Autodesk Inventor part; units mm, degrees
ref_plane "YZ Plane" through (0, 0, 0) normal (1, 0, 0) x (0, 1, 0)
ref_plane "XZ Plane" through (0, 0, 0) normal (0, 1, 0) x (-1, 0, 0)
ref_plane "XY Plane" through (0, 0, 0) normal (0, 0, 1) x (1, 0, 0)
sketch "Sketch1" plane through (0, 0, 0) normal (0, 1, 0) x (-1, 0, 0)
  line L0 (17.6552, 44.8276) -> (77.6552, 44.8276)
  line L1 (77.6552, 44.8276) -> (77.6552, -15.1724)
  line L2 (77.6552, -15.1724) -> (17.6552, -15.1724)
  line L3 (17.6552, -15.1724) -> (17.6552, 44.8276)
  point P0 (0, 0)
  dimension "d0" = 60
  dimension "d1" = 60
extrude "Extrusion1" add sketch "Sketch1" along normal blind 25
sketch "Sketch2" plane through (0, 25, 0) normal (0, 1, 0) x (1, 0, 0)
  line L0 (-17.6552, -44.8276) -> (-17.6552, 15.1724)
  line L1 (-17.6552, 15.1724) -> (-77.6552, 15.1724)
  line L2 (-77.6552, 15.1724) -> (-77.6552, -44.8276)
  circle A0 centre (-47.6552, -14.8276) radius 26
  circle A1 centre (-73.6552, 11.1724) radius 2.15
  circle A2 centre (-21.6552, 11.1724) radius 2.15
  circle A3 centre (-21.6552, -40.8276) radius 2.15
  circle A4 centre (-73.6552, -40.8276) radius 2.15
  point P0 (0, 0)
  dimension "d4" = 52
  dimension "d5" = 30
  dimension "d6" = 30
  dimension "d7" = 4.3
  dimension "d8" = 4.3
  dimension "d9" = 4.3
  dimension "d10" = 4.3
  dimension "d11" = 52
  dimension "d12" = 52
  dimension "d13" = 52
  dimension "d14" = 52
  dimension "d15" = 4
  dimension "d16" = 4
  dimension "d17" = 4
  dimension "d18" = 4
extrude "Extrusion2" cut sketch "Sketch2" against normal blind 38
properties part number "Fan60"
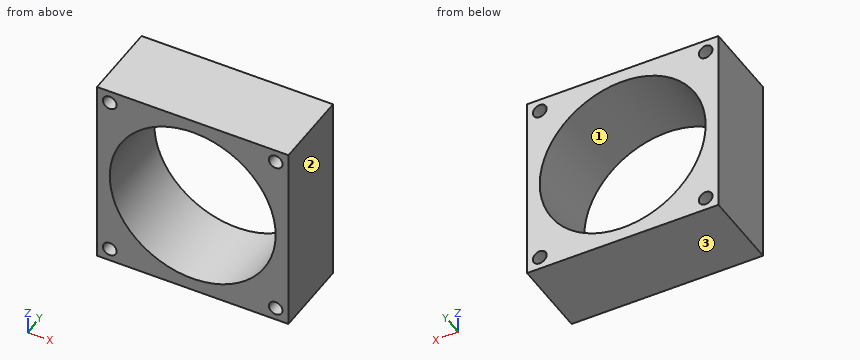
Source: CAD feature listing. Evaluate the final solid. Frame: model axes, mm. Face numbers are marked on the shaded views. Round coordinates to 2 decimals unless told otherwise and drop trailing zeros. Write each loop counter-clockwise with the first axis right and the second up, starting at its lowest first coordinate (ties: lowest second). Pieces come first, ordered by that corner, then holes. Notation, with made-up numbers: M -37,70 L -7,70 A10 cw -7,79 Z; hole C -10.75,28 d9. An arc over 180 degrees is marked long. Use CSV: the item, a comma, the result in double quotes. Start each with the question number.
Q1. Line query: line 1 (Z direction, x = -21.5, y = 5.75); line 2 (Z direction, x = -20, y = 4); line 3 (Z direction, x = -45, y = 19). Output: solid intervals per line, ascending. Write a range as from..to.
Q2. Cut plane C-C on y = 22.25. Output: boundary loops of the cut face in (x, z), plus the area to 3 significant figures.
Q3. Cut plane A-A on x = -59. Output: boundary loops of the cut face in (y, z).
Q4. Pull-direction query (X, two-part tool) for the marked faces 1, 2 and 3; classes: +X half, -X half, draft (parallel to the pull), parting line (faces both ways), or undercut.
Q5. First-contact query: P1, Ø8, axis at x = -42.5, z = -3, coming from the +Y side. Flat tip, straight axial feed; report the tip coordinate or a pass-through.
Q6. Cut plane B-B on z = 32. Output: boundary loops of the cut face in (x, y).
Results found:
1,line 1,"-15.17..-13.32, -9.03..38.68, 42.97..44.83"
1,line 2,"-15.17..-12.54, -9.8..39.46, 42.2..44.83"
1,line 3,"-15.17..-11.04, 40.69..44.83"
2,outline,"M -77.66,-15.17 L -17.66,-15.17 L -17.66,44.83 L -77.66,44.83 Z; hole C -73.66,-11.17 d4.3; hole C -73.66,40.83 d4.3; hole C -47.66,14.83 d52; hole C -21.66,-11.17 d4.3; hole C -21.66,40.83 d4.3"
2,area,"1,420 mm^2"
3,outline,"M 0,-15.17 L 25,-15.17 L 25,-8.57 L 0,-8.57 Z; M 0,38.22 L 25,38.22 L 25,44.83 L 0,44.83 Z"
4,face 1,"undercut"
4,face 2,"+X half"
4,face 3,"draft"
5,P1,"through"
6,outline,"M -77.66,0 L -67.18,0 L -67.18,25 L -77.66,25 Z; M -28.13,0 L -17.66,0 L -17.66,25 L -28.13,25 Z"
